Work out the finished part from the listing and answer in its coordinate system (mm). A direction names the side the tool comes from. Round coordinates to 2 decimals unless told otherwise and drop trailing zeros. Order: outer loops, then holes, each group sorted by start corner. A loop starts at its lowest first (then second) coordinate and runs counter-clockwise, first axis right, second up. Notation, with made-up numbers: (50.25, 80) -> (61.25, 80) arc R26 cw to (61.25, 118) -> close; hole circle Ø11 at (-38.75, 52.5). An arc over 180 degrees is marked (long way). Use one line per item in the form item = value.
```python
from build123d import *

# Parameters (mm, degrees)
SKETCH1_W           = 55
SKETCH1_H           = 38
SKETCH1_R           = 0.9
BOSS_EXTRUDE1_DEPTH = 0.75
SKETCH2_W           = 33.4
SKETCH2_H           = 17.4
BOSS_EXTRUDE2_DEPTH = 2.4
SKETCH4_W           = 6.275
SKETCH4_H           = 3.5
BOSS_EXTRUDE3_DEPTH = 1.85
SKETCH6_W           = 3
SKETCH6_H           = 1.6
BOSS_EXTRUDE4_DEPTH = 0.45


with BuildPart() as part:
    # Sketch1 → Boss-Extrude1 (new, symmetric)
    with BuildSketch(Plane.XY):
        Rectangle(SKETCH1_W, SKETCH1_H)
        with Locations((25.6, 17.1)):
            Circle(SKETCH1_R, mode=Mode.SUBTRACT)
        with Locations(Location((-25.6, 17.1, 0), (0, 0, 180))):
            Circle(SKETCH1_R, mode=Mode.SUBTRACT)
        with Locations(Location((25.6, -17.1, 0), (0, 0, 180))):
            Circle(SKETCH1_R, mode=Mode.SUBTRACT)
        with Locations((-25.6, -17.1)):
            Circle(SKETCH1_R, mode=Mode.SUBTRACT)
    extrude(amount=BOSS_EXTRUDE1_DEPTH, both=True)

    # Sketch2 → Boss-Extrude2 (add, symmetric)
    with BuildSketch(Plane.XY.offset(0.75)):
        with Locations((-1.3, 6.2)):
            Rectangle(SKETCH2_W, SKETCH2_H)
    extrude(amount=BOSS_EXTRUDE2_DEPTH, both=True)

    # Sketch4 → Boss-Extrude3 (add, symmetric)
    with BuildSketch(Plane.XY.offset(0.75)):
        with Locations((18.7125, -16.25)):
            Rectangle(SKETCH4_W, SKETCH4_H)
        with Locations((-18.1125, -16.25)):
            Rectangle(SKETCH4_W, SKETCH4_H)
        with Locations((6.8375, -16.25)):
            Rectangle(SKETCH4_W, SKETCH4_H)
        with Locations((-5.0375, -16.25)):
            Rectangle(SKETCH4_W, SKETCH4_H)
        with Locations((-18.1125, -11.75)):
            Rectangle(SKETCH4_W, SKETCH4_H)
        with Locations((-5.0375, -11.75)):
            Rectangle(SKETCH4_W, SKETCH4_H)
        with Locations((6.8375, -11.75)):
            Rectangle(SKETCH4_W, SKETCH4_H)
        with Locations((18.7125, -11.75)):
            Rectangle(SKETCH4_W, SKETCH4_H)
    extrude(amount=BOSS_EXTRUDE3_DEPTH, both=True)

    # Sketch6 → Boss-Extrude4 (add, symmetric)
    with BuildSketch(Plane.XY.offset(2.6)):
        with Locations((18.7125, -16.25)):
            Rectangle(SKETCH6_W, SKETCH6_H)
        with Locations((6.9125, -16.25)):
            Rectangle(SKETCH6_W, SKETCH6_H)
        with Locations((-4.8875, -16.25)):
            Rectangle(SKETCH6_W, SKETCH6_H)
        with Locations((6.9125, -11.75)):
            Rectangle(SKETCH6_W, SKETCH6_H)
        with Locations((-4.8875, -11.75)):
            Rectangle(SKETCH6_W, SKETCH6_H)
        with Locations((18.7125, -11.75)):
            Rectangle(SKETCH6_W, SKETCH6_H)
        with Locations((-18.1375, -16.25)):
            Rectangle(SKETCH6_W, SKETCH6_H)
        with Locations((-18.1375, -11.75)):
            Rectangle(SKETCH6_W, SKETCH6_H)
    extrude(amount=BOSS_EXTRUDE4_DEPTH, both=True)


solid = part.part
```
Item 1: For faces 4 (the flat face through (7, -16, -1.1)), 5 (the flat face through (-2, -2.5, 2)), 6 (the flat face through (-2, 14.9, 2)), 7 (the flat face through (15.575, -16, 2)), 8 (the flat face through (15.4, 6, 2)), determine the directions among +Z, -Z, +X, -X, +Y, -Y from which every point of the face is accessible in a straight line to the end or side of a thin tool.
Findings:
face_4 = -Z, +X, -X, -Y
face_5 = +Z, +X, -X
face_6 = +Z, +X, -X, +Y
face_7 = +Z, +Y, -Y
face_8 = +Z, +X, +Y, -Y
Item 2: Determine the mould class of faces 1 (the flat face through (7, -16, 3.05)), 2 (the flat face through (-18, -15, 2.6)), 3 (the flat face through (0, -19, 0)) for opening direction Y: released by +Y, released by -Y, zero draft, split by the parting line, or undercut.
Findings:
face_1 = zero draft
face_2 = undercut
face_3 = released by -Y
Item 3: The part is cut by section D-D, the plane x = 13. Give the vertices of the cut face in (y, z).
Findings:
outline = (-19, -0.75) -> (-2.5, -0.75) -> (-2.5, -1.65) -> (14.9, -1.65) -> (14.9, -0.75) -> (19, -0.75) -> (19, 0.75) -> (14.9, 0.75) -> (14.9, 3.15) -> (-2.5, 3.15) -> (-2.5, 0.75) -> (-19, 0.75) -> close
Item 4: The part is cut by section C-C, the plane y = 5. Give the vertices of the cut face in (x, z).
Findings:
outline = (-27.5, -0.75) -> (-18, -0.75) -> (-18, -1.65) -> (15.4, -1.65) -> (15.4, -0.75) -> (27.5, -0.75) -> (27.5, 0.75) -> (15.4, 0.75) -> (15.4, 3.15) -> (-18, 3.15) -> (-18, 0.75) -> (-27.5, 0.75) -> close
Item 5: Consider line 1 along Y through (x, z) = (25.6, 0.45); line 2 along Y through (x, z) = (-3, 2.25); line 3 along Z through (x, y) = (12, -13.5). Determine where each line is inside the solid, lowest interval first.
Findings:
line_1 = -19 to -18, -16.2 to 16.2, 18 to 19
line_2 = -18 to -14.5, -13.5 to -10, -2.5 to 14.9
line_3 = -0.75 to 0.75
Item 6: The part is cut by section A-A, the plane x = -25.6. Give the vertices of the cut face in (y, z).
Findings:
outline = (-19, -0.75) -> (-18, -0.75) -> (-18, 0.75) -> (-19, 0.75) -> close; (-16.2, -0.75) -> (16.2, -0.75) -> (16.2, 0.75) -> (-16.2, 0.75) -> close; (18, -0.75) -> (19, -0.75) -> (19, 0.75) -> (18, 0.75) -> close
Item 7: Flat-ended cylindrical pins translate along their axes: P1, Ø0.8, axis at x = -4.5, y = -16.5, coming from the +Z side; P2, Ø0.5, axis at y = -16.5, z = 3, coming from the +X side; P3, Ø0.9, axis at x = -6.5, z = 2, coming from the -Y side. Find the tip coordinate at first contact, or state that the pin passes through.
Findings:
P1 = 3.05
P2 = 20.21
P3 = -18
Item 8: The part is cut by section B-B, the plane y = 17.1. Give the vertices of the cut face in (x, z).
Findings:
outline = (-27.5, -0.75) -> (-26.5, -0.75) -> (-26.5, 0.75) -> (-27.5, 0.75) -> close; (-24.7, -0.75) -> (24.7, -0.75) -> (24.7, 0.75) -> (-24.7, 0.75) -> close; (26.5, -0.75) -> (27.5, -0.75) -> (27.5, 0.75) -> (26.5, 0.75) -> close
